Source: CAD feature listing. Evaluate the final solid. Frame: model axes, mm. A direction names the side the tool comes from. Give positions to 0.01 mm unless a question says otherwise; leave off trailing zeros. Write each loop counter-clockwise with the first axis right and the second up, starting at its lowest first coordinate (ties: lowest second). Pieces come first, ordered by that corner, then holes. Notation, with made-up numbers: M 63,71 L 110,71 A24 ccw 110,94 Z; hole C 86.5,-38.75 d8. An arc over 180 degrees is marked long. Return JSON: item names as keys, results as strings.
```python
from build123d import *

# Parameters (mm, degrees)
SKETCH3_W   = 14.319236131
SKETCH3_H   = 126.612193163
SKETCH3_W_2 = 30.145760277
SKETCH3_H_2 = 185.396425703
SKETCH3_W_3 = 12.058304111
SKETCH3_H_3 = 222.324982043


with BuildPart() as part:
    # Sketch2 → Revolve1 (revolve)
    with BuildSketch(Plane(origin=(0, 0, 0), x_dir=(0, 0, -1), z_dir=(1, 0, 0)), mode=Mode.PRIVATE) as revolve1_sk:
        with BuildLine():
            Line((-33.902439024, 170), (-33.902439024, 130))
            Line((-33.902439024, 130), (26.097560976, 130))
            Line((26.097560976, 130), (26.097560976, 170))
            ThreePointArc((26.097560976, 170), (-3.902439024, 200), (-33.902439024, 170))
        make_face()
    revolve(revolve1_sk.sketch.rotate(Axis((0, 0, 102.578397213), (0, 0, -1)), 90), axis=Axis((0, 0, 102.578397213), (0, 0, -1)))

    # Sketch3 → Cut-Revolve1 (revolve, cut)
    with BuildSketch(Plane(origin=(0, 0, 0), x_dir=(0, 0, -1), z_dir=(1, 0, 0)), mode=Mode.PRIVATE) as cut_revolve1_sk:
        with Locations((-4.789385206, 256.956129248)):
            Rectangle(SKETCH3_W, SKETCH3_H)
        with Locations((-33.804679472, 280.695915466)):
            Rectangle(SKETCH3_W_2, SKETCH3_H_2)
        with Locations((14.428536971, 299.160193636)):
            Rectangle(SKETCH3_W_3, SKETCH3_H_3)
    revolve(cut_revolve1_sk.sketch.rotate(Axis((0, 0, 101.363868033), (0, 0, -1)), 90), axis=Axis((0, 0, 101.363868033), (0, 0, -1)), mode=Mode.SUBTRACT)


solid = part.part
```
1) Contact query for flat-ended pins moving along their axis: pin 1 Ø8 at (x, z) = (-64, 23.5) entering from -Y; pin 2 Ø6 at (y, z) = (-47, 11.5) entering from +X; pin 3 Ø1.5 at (y, z) = (-113.5, 26.5) entering from +X. Output: stop coordinate, or through.
Numbers:
{"pin 1": "stops at y = -178.17", "pin 2": "stops at x = 193.97", "pin 3": "stops at x = 150.43"}
2) Draft query along Z for faces 1 (the face through (123.997, -39.048, 3.482)), 2 (the face through (-43, 191, 11.949)), 3 (the face through (-175, 72, -8.399)). Return one class per face: released by +Z, released by -Z, zero draft, split by the parting line, or undercut.
Numbers:
{"face 1": "zero draft", "face 2": "undercut", "face 3": "released by -Z"}
3) Set-up query: faces 4 (the face through (101.1, -158.5, -14.3)), 5 (the face through (-159, 101, 18.732)), 6 (the face through (163.4, -104.3, -2.37)), 7 (the face through (39, 125, -26.098)). Return all of +Z, -Z, +X, -X, +Y, -Y with unobstructed straight access to the full face (end or side cutting, diameter ignored); none if empty.
Numbers:
{"face 4": "-Z", "face 5": "+Z", "face 6": "none", "face 7": "-Z, +X, -X, +Y, -Y"}
4) Cut plane A-A, the plane x = 0. Return the cut outline in (y, z).
Numbers:
{"outline": "M -199.34,-2.37 A30 ccw -197.36,-8.4 L -188,-8.4 L -188,-20.1 A30 ccw -170,-26.1 L -130,-26.1 L -130,33.9 L -170,33.9 A30 ccw -188,27.9 L -188,18.73 L -196.08,18.73 A30 ccw -198.9,11.95 L -193.65,11.95 L -193.65,-2.37 Z; M 130,-26.1 L 170,-26.1 A30 ccw 188,-20.1 L 188,-8.4 L 197.36,-8.4 A30 ccw 199.34,-2.37 L 193.65,-2.37 L 193.65,11.95 L 198.9,11.95 A30 ccw 196.08,18.73 L 188,18.73 L 188,27.9 A30 ccw 170,33.9 L 130,33.9 Z"}
5) Line query: line 1 (Y direction, x = 0, z = 9); line 2 (Y direction, x = 0, z = 20.5); line 3 (Z direction, x = 143.5, y = -136). Output: solid intervals per line, ascending. Write a range as [from, to].
Numbers:
{"line 1": "y = [-193.65, -130], [130, 193.65]", "line 2": "y = [-188, -130], [130, 188]", "line 3": "z = [-7.6, -2.37], [11.95, 15.4]"}
